Geometry: final body of the model. Coordinates: model frame, mm. A direction names the side the tool comes from. Give positions to 0.01 mm unless a question says otherwise; leave off trailing zeros. Loops run counter-clockwise (first coordinate to the right, second up) from the corner with the lowest first, then second, coordinate; pieces in that order, holes last. Notation, with made-up numbers: (19.25, 60) -> (54.25, 60) arc R19 ccw to (54.25, 84) -> close; hole circle Ø11 at (-17.75, 51). An arc over 180 degrees is marked (long way). Answer in a Markdown table with one row per item. Add a question column.
Autodesk Inventor part; units mm, degrees
ref_plane "Work Plane1" through (0, 5, 0) normal (0, 1, 0) x (-1, 0, 0)
ref_plane "YZ Plane" through (0, 0, 0) normal (1, 0, 0) x (0, 1, 0)
ref_plane "XZ Plane" through (0, 0, 0) normal (0, 1, 0) x (-1, 0, 0)
sketch "Sketch1" plane through (0, 0, 0) normal (0, 1, 0) x (-1, 0, 0)
  line L0 (0, 0) -> (4.0002, 0)
  line L1 (4.0002, 0) -> (5, -0.9998)
  line L2 (5, -0.9998) -> (5, -8)
  line L3 (5, -8) -> (4.5, -8)
  line L4 (4.5, -8) -> (4.5, -9.5)
  line L5 (4.5, -9.5) -> (5, -9.5)
  line L6 (5, -9.5) -> (5, -76.5)
  line L7 (5, -76.5) -> (4.5, -76.5)
  line L8 (4.5, -76.5) -> (4.5, -78)
  line L9 (4.5, -78) -> (5, -78)
  line L10 (5, -78) -> (5, -79)
  line L11 (5, -79) -> (4, -80)
  line L12 (4, -80) -> (0, -80)
  line L13 (0, -80) -> (0, 0)
  dimension "d9" = 80
  dimension "d10" = 5
  dimension "d11" = 0.5
  dimension "d12" = 1.5
  dimension "d13" = 1.5
  dimension "d14" = 2
  dimension "d15" = 1
  dimension "d16" = 135
  dimension "d17" = 67
  dimension "d18" = 135
  dimension "d19" = 1.414
revolve "Revolution1" add sketch "Sketch1" angle 360 about axis through (0, 0, -80) along (0, 0, 1)
sketch "Sketch2" plane through (0, 0, 0) normal (0, 0, 1) x (1, 0, 0)
  circle A0 centre (0, 0) radius 3
  dimension "d21" = 6
extrude "Extrusion1" cut sketch "Sketch2" against normal blind 10
ref_plane "Work Plane1" through (0, 5, 0) normal (0, 1, 0) x (-1, 0, 0)
sketch "Sketch3" plane through (0, 5, 0) normal (0, 1, 0) x (-1, 0, 0)
  line L0 (-5, -9.5) -> (5, -9.5)
  line L1 (-5, -76.5) -> (5, -76.5)
  line L2 (-5, -9.5) -> (-5, -76.5)
  line L3 (5, -9.5) -> (5, -76.5)
  circle A0 centre (0, -43) radius 2.5
  point P0 (0, 0)
  dimension "d25" = 5
  dimension "d26" = 67
  dimension "d27" = 33.5
extrude "Extrusion2" cut sketch "Sketch3" against normal blind 10 contours A0
sketch "Sketch4" plane through (0, 5, 0) normal (0, 1, 0) x (-1, 0, 0)
  line L0 (-5, -0.9998) -> (5, -0.9998)
  line L1 (-5, -8) -> (5, -8)
  line L2 (-5, -0.9998) -> (-5, -8)
  line L3 (5, -0.9998) -> (5, -8)
  circle A0 centre (0, -4) radius 1.5
  line L4 (-4.0002, 0) -> (4.0002, 0)
  point P0 (0, 0)
  dimension "d30" = 3
  dimension "d31" = 4
extrude "Extrusion3" cut sketch "Sketch4" against normal up to surface contours A0
thread "Thread1"
thread "Thread2"
equation "\"d27\" = 0.5 * d26"
properties part number "potentiometer_aksel"
(1) Draft query along Y for faces 1 (the cylindrical face through (-0.65, -2.93, -4.93)), 2 (the cylindrical face through (-2.31, 0.07, -43.96)), 3 (the cylindrical face through (-3, 4, -43)). Return one class per face: +Y half, -Y half, draft (parallel to the pull), parting line (faces both ways), or undercut.
(2) Pin query (flat end, axial travel): pin 1 Ø1.5 at (x, z) = (2, -42.5) entering from +Y. Return the tip coordinate at first contact, or that it passes through.
(3) Cut plane C-C on x = 0. State how many separate pieces and enclosed holes the cut face has, then the cut area to 3 significant figures.
(4) Cut plane B-B on z = -6.5. Return the cut outline in (x, y), then the cut area to 3 significant figures.
(5) Reachability of faces 4 (the flat face through (-1, -3, 0)), 5 (the flat face through (0, 0, -10)), 6 (the cylindrical face through (-1.43, 3.82, -3.55)), 7 (the cylindrical face through (0.59, 4.46, -8.76)), 8 (the cylindrical face through (1.08, -4.88, -78.51)) from +Z, -Z, +X, -X, +Y, -Y: full face, straight path, thin tool, end or side. Return the list, or none.
(6) Cut plane D-D on z = -43. Return the cut outline in (x, y), then the cut area to 3 significant figures.
(7) Material intervals for line 1 along Z through (x, y) = (0, 3.4); line 2 along Y through (x, z) = (0, -7.5); line 3 along Y through (x, z) = (-0.25, -35.5), sorted ascending. Write a range as from..to.
Answer list:
| question | item | result |
|---|---|---|
| 1 | face 1 | undercut |
| 1 | face 2 | draft |
| 1 | face 3 | parting line |
| 2 | pin 1 | stops at y = 4.5 |
| 3 | separate pieces | 3 |
| 3 | enclosed holes | 0 |
| 3 | area | 679 mm² |
| 4 | outline | circle Ø10 at (0, 0); hole circle Ø6 at (0, 0) |
| 4 | area | 50.3 mm² |
| 5 | face 4 | +Z, +X, -X, +Y, -Y |
| 5 | face 5 | +Z |
| 5 | face 6 | +Y |
| 5 | face 7 | none |
| 5 | face 8 | +Z, -Z |
| 6 | outline | (-2.5, -4.33) -> (-2.5, 4.33) arc R5 ccw to start; (2.5, -4.33) arc R5 ccw to (2.5, 4.33) -> close |
| 6 | area | 30.7 mm² |
| 7 | line 1 | z = -80..-45.5, -40.5..-5.5, -2.5..0 |
| 7 | line 2 | y = -5..-3, 3..5 |
| 7 | line 3 | y = -4.99..4.99 |
